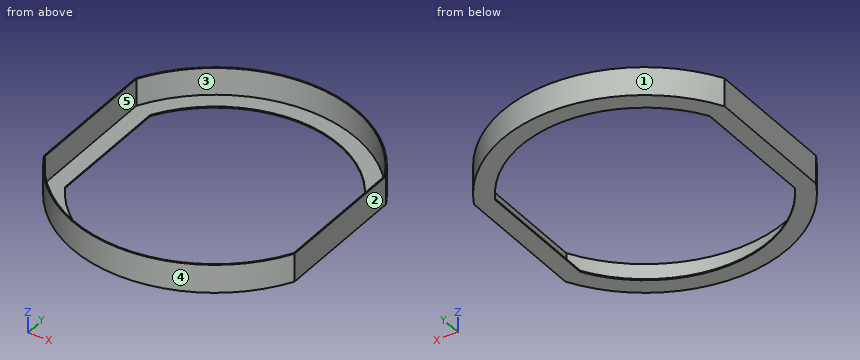
Autodesk Inventor part; units mm, degrees
ref_plane "YZ Plane" through (0, 0, 0) normal (1, 0, 0) x (0, 1, 0)
ref_plane "XZ Plane" through (0, 0, 0) normal (0, 1, 0) x (-1, 0, 0)
ref_plane "XY Plane" through (0, 0, 0) normal (0, 0, 1) x (1, 0, 0)
sketch "Sketch1" plane through (0, 0, 0) normal (0, 0, 1) x (1, 0, 0)
  arc A0 (22, 11.8743) -> (-22, 11.8743) centre (0, 0) ccw
  arc A1 (-22, -11.8743) -> (22, -11.8743) centre (0, 0) ccw
  line L0 (-22, 11.8743) -> (-22, -11.8743)
  line L1 (22, -11.8743) -> (22, 11.8743)
  line L2 (-22.2, 11.9248) -> (-22.2, -11.9248)
  arc A2 (-22.2, -11.9248) -> (22.2, -11.9248) centre (0, 0) ccw
  line L3 (22.2, -11.9248) -> (22.2, 11.9248)
  arc A3 (22.2, 11.9248) -> (-22.2, 11.9248) centre (0, 0) ccw
  line L4 (-19, 11.0905) -> (-19, -11.0905)
  arc A4 (-19, -11.0905) -> (19, -11.0905) centre (0, 0) ccw
  line L5 (19, -11.0905) -> (19, 11.0905)
  arc A5 (19, 11.0905) -> (-19, 11.0905) centre (0, 0) ccw
  point P0 (-22, 0)
  point P1 (22, 0)
  dimension "d1" = 44
  dimension "d2" = 50
  dimension "d3" = 3
  dimension "d4" = 0.2
extrude "Extrusion1" add sketch "Sketch1" along normal blind 0.2 contours L1 A1 L0 A0
extrude "Extrusion2" add sketch "Sketch1" along normal blind 5 contours A3 L3 A2 L2
equation "\"d4\" = thickness"
equation "\"d5\" = thickness"
equation "\"thickness\" = 0.2"
properties part number "probe-gate-mesh" material "Stainless Steel"
Geometry check sheet. Reference: the model listing, model coordinates, mm. Face numbers are marked on the shaded views. A direction names the side the tool comes from. Coordinates: 2 decimals unless noted, no trailing zeros. Order: outer loops, then holes, each group sorted by start corner. A loop starts at its lowest first (then second) coordinate and runs counter-clockwise, first axis right, second up. Notation, with made-up numbers: (-13.75, -28.75) - (-4.75, -28.75) arc R14 cw to (-4.75, -3.75) - close; hole circle Ø5 at (58, 80). An arc over 180 degrees is marked (long way). Answer in a Markdown table with one row per item. Add a question column.
1. Draft check along Y on the marked faces 1, 2 and 3. Enter one of: +Y half, -Y half, draft (parallel to the pull), parting line (faces both ways), or undercut.
2. Section check B-B (x = -16.5). Enter the section's corners in (y, z), plus the area to 3 significant figures.
3. Access from +Z, -Z, +X, -X, +Y, -Y to the whole of each face (thin tool, end or side, straight path). Record for the marked faces 4 and 5.
4. Section check C-C (y = 3.5). Enter the section's corners in (x, z), plus the area to 3 significant figures.
5. Section check A-A (z = 2.15). Enter the section's corners in (x, y), plus the area to 3 significant figures.
6. Material ranges on L1, parallel to X at y = 3, z = 4.8; L2, parallel to Y at x = -12, z = 3.95; L3, parallel to X at y = 17, z = 1.05, recorded low to high. Write a range as [from, to].
7. Gauge pin test, flat ends, axial feed: pin 1 Ø1 at (x, z) = (4, 3) entering from +Y; pin 2 Ø3 at (x, z) = (16.5, 2) entering from +Y; pin 3 Ø1.5 at (x, z) = (6.5, 3) entering from -Y. Record the tip position at first contact, or that the pin passes through.
Data:
| question | item | result |
|---|---|---|
| 1 | face 1 | +Y half |
| 1 | face 2 | draft |
| 1 | face 3 | undercut |
| 2 | outline | (-19.05, 0) - (-14.55, 0) - (-14.55, 0.2) - (-18.78, 0.2) - (-18.78, 5) - (-19.05, 5) - close; (14.55, 0) - (19.05, 0) - (19.05, 5) - (18.78, 5) - (18.78, 0.2) - (14.55, 0.2) - close |
| 2 | area | 4.35 mm² |
| 3 | face 4 | +Z, -Z, -Y |
| 3 | face 5 | +Z |
| 4 | outline | (-22.2, 0) - (-19, 0) - (-19, 0.2) - (-22, 0.2) - (-22, 5) - (-22.2, 5) - close; (19, 0) - (22.2, 0) - (22.2, 5) - (22, 5) - (22, 0.2) - (19, 0.2) - close |
| 4 | area | 3.20 mm² |
| 5 | outline | (-22.2, -11.92) arc R25.2 ccw to (22.2, -11.92) - (22.2, 11.92) arc R25.2 ccw to (-22.2, 11.92) - close; hole (-22, -11.87) arc R25 ccw to (22, -11.87) - (22, 11.87) arc R25 ccw to (-22, 11.87) - close |
| 5 | area | 31.1 mm² |
| 6 | L1 | x = [-22.2, -22], [22, 22.2] |
| 6 | L2 | y = [-22.16, -21.93], [21.93, 22.16] |
| 6 | L3 | x = [-18.6, -18.33], [18.33, 18.6] |
| 7 | pin 1 | stops at y = 24.96 |
| 7 | pin 2 | stops at y = 20.25 |
| 7 | pin 3 | stops at y = -24.54 |
